```python
from build123d import *

# Parameters (mm, degrees)
SKETCH2_R           = 28.5
SKETCH2_R_2         = 22.6
BOSS_EXTRUDE1_DEPTH = 62
CHAMFER1_SIZE       = 2
CHAMFER2_SIZE       = 1
CHAMFER3_SIZE       = 1


with BuildPart() as part:
    # Sketch2 → Boss-Extrude1 (new body)
    with BuildSketch(Plane(origin=(0, 0, 0), x_dir=(1, 0, 0), z_dir=(0, 1, 0))):
        with Locations(Location((0, 0, 0), (0, 0, 270))):
            Circle(SKETCH2_R)
        with Locations(Location((0, 0, 0), (0, 0, 270))):
            Circle(SKETCH2_R_2, mode=Mode.SUBTRACT)
    extrude(amount=BOSS_EXTRUDE1_DEPTH)

    # Chamfer1
    chamfer1_edges = [part.edges().sort_by_distance(p)[0] for p in [
        (0, 62, -22.6),
    ]]
    chamfer(chamfer1_edges, length=CHAMFER1_SIZE)

    # Chamfer2
    chamfer2_edges = [part.edges().sort_by_distance(p)[0] for p in [
        (0, 0, -22.6),
    ]]
    chamfer(chamfer2_edges, length=CHAMFER2_SIZE)

    # Chamfer3
    chamfer3_edges = [part.edges().sort_by_distance(p)[0] for p in [
        (0, 0, -28.5),
    ]]
    chamfer(chamfer3_edges, length=CHAMFER3_SIZE)


solid = part.part
```
Geometry check sheet. Reference: the model listing, model coordinates, mm. Coordinates: 2 decimals unless noted, no trailing zeros. Loops run counter-clockwise (first coordinate to the right, second up) from the corner with the lowest first, then second, coordinate; pieces in that order, holes last. Notation, with made-up numbers: (-20, 38.5) - (22, 38.5) arc R28 cw to (22, 72.5) - close; hole circle Ø1 at (1.5, 58). An arc over 180 degrees is marked (long way). One line per item, written item: value. Start each with the question number.
(1) Material ranges on line 1 (X direction, y = 18.5, z = 0); line 2 (Z direction, x = -11, y = 10); line 3 (Z direction, x = 3, y = 3), recorded low to high. Write a range as [from, to].
(2) Depth check by flat-ended pin: P1, Ø1.5, axis at y = 40.5, z = 6, coming from the +X side; P2, Ø5, axis at y = 47, z = -22.5, coming from the +X side; P3, Ø8, axis at x = 19, z = -17.5, coming from the -Y side; P4, Ø4, axis at y = 45.5, z = 0, coming from the +X side. Enter the tip coordinate at first touch or a pass-through.
(3) Mould release check, pull along Z, two halves, no side actions. Record for faces 1 (the cylindrical face through (-27.82, 31.07, -6.18)), 2 (the flat face through (-8.3, 62, -23.4)), 3 (the conical face through (6.83, 60.13, 21.68)): released by +Z, released by -Z, zero draft, split by the parting line, or undercut.
(4) Cross-section at C-C on y = 43. Enter the section's corners in (x, z).
(5) Cross-section at B-B on z = 0. Enter the section's corners in (x, y), plus the area to 3 significant figures.
(6) Cross-section at A-A on x = 0. Enter the section's corners in (y, z).
Results below:
1. line 1: x = [-28.5, -22.6], [22.6, 28.5]
1. line 2: z = [-26.29, -19.74], [19.74, 26.29]
1. line 3: z = [-28.34, -22.4], [22.4, 28.34]
2. P1: stops at x = 28.01
2. P2: stops at x = 20.3
2. P3: stops at y = 0
2. P4: stops at x = 28.5
3. face 1: split by the parting line
3. face 2: zero draft
3. face 3: undercut
4. outline: circle Ø57 at (0, 0); hole circle Ø45.2 at (0, 0)
5. outline: (-28.5, 1) - (-27.5, 0) - (-23.6, 0) - (-22.6, 1) - (-22.6, 60) - (-24.6, 62) - (-28.5, 62) - close; (22.6, 1) - (23.6, 0) - (27.5, 0) - (28.5, 1) - (28.5, 62) - (24.6, 62) - (22.6, 60) - close
5. area: 726 mm2
6. outline: (0, -27.5) - (1, -28.5) - (62, -28.5) - (62, -24.6) - (60, -22.6) - (1, -22.6) - (0, -23.6) - close; (0, 23.6) - (1, 22.6) - (60, 22.6) - (62, 24.6) - (62, 28.5) - (1, 28.5) - (0, 27.5) - close
